For this review, take the finished solid that the model builds, in its own axes (mm). Give positions to 0.01 mm unless a question says otherwise; leave off trailing zeros. Order: outer loops, then holes, each group sorted by start corner. A loop starts at its lowest first (then second) coordinate and runs counter-clockwise, first axis right, second up. Notation, with made-up numbers: (88, 39.5) - (136, 39.5) arc R28 ccw to (136, 77.5) - close; hole circle Ø6 at (-21.75, 73). An arc over 180 degrees is marked (long way). Use a Markdown table: item, result. Add a question column.
1) We need section A-A on y = 2.05. Write out the cut boundary in (x, z), then the cut area to 4 significant figures.
2) Wall thickness on L1, parallel to Z at x = 0.4, y = 3.6; L2, parallel to Z at x = 2.8, y = 2.15; L3, parallel to Y at x = 2.05, z = 62: over which ranges is each line inside the solid? List them lowest first.
3) We need section B-B on x = 2.3. Write out the cut boundary in (y, z).
4) Clearance check with flat-ended pins moving along their axes: P1, Ø1, axis at x = 3, z = 26.5, coming from the -Y side; P2, Ø1.2, axis at x = 2.5, z = 129.5, coming from the +Y side; P3, Ø0.8, axis at x = 2.5, z = 130.5, coming from the -Y side; P4, Ø0.8, axis at y = 2, z = -1.5, coming from the -X side. State where each tip first meets the part, or that it passes through.
```python
from build123d import *

# Parameters (mm, degrees)
SKETCH1_W           = 5
SKETCH1_H           = 5
BOSS_EXTRUDE1_DEPTH = 127.3
SKETCH2_W           = 2.5
SKETCH2_H           = 2.5
BOSS_EXTRUDE2_DEPTH = 5
SKETCH3_W           = 2.5
SKETCH3_H           = 2.5
BOSS_EXTRUDE3_DEPTH = 5
SKETCH4_W           = 3
SKETCH4_H           = 3
CUT_EXTRUDE1_DEPTH  = 30


with BuildPart() as part:
    # Sketch1 → Boss-Extrude1 (new body)
    with BuildSketch(Plane.XY):
        with Locations((2.5, 2.5)):
            Rectangle(SKETCH1_W, SKETCH1_H)
    extrude(amount=BOSS_EXTRUDE1_DEPTH)

    # Sketch2 → Boss-Extrude2 (add)
    with BuildSketch(Plane(origin=(0, 0, 0), x_dir=(-1, 0, 0), z_dir=(0, 0, -1))):
        with Locations((-2.5, 2.5)):
            Rectangle(SKETCH2_W, SKETCH2_H)
    extrude(amount=BOSS_EXTRUDE2_DEPTH)

    # Sketch3 → Boss-Extrude3 (add)
    with BuildSketch(Plane.XY.offset(127.3)):
        with Locations((2.5, 2.5)):
            Rectangle(SKETCH3_W, SKETCH3_H)
    extrude(amount=BOSS_EXTRUDE3_DEPTH)

    # Sketch4 → Cut-Extrude1 (cut)
    with BuildSketch(Plane.ZY):
        with Locations((61.15, 2.5)):
            Rectangle(SKETCH4_W, SKETCH4_H)
    extrude(amount=-CUT_EXTRUDE1_DEPTH, mode=Mode.SUBTRACT)


solid = part.part
```
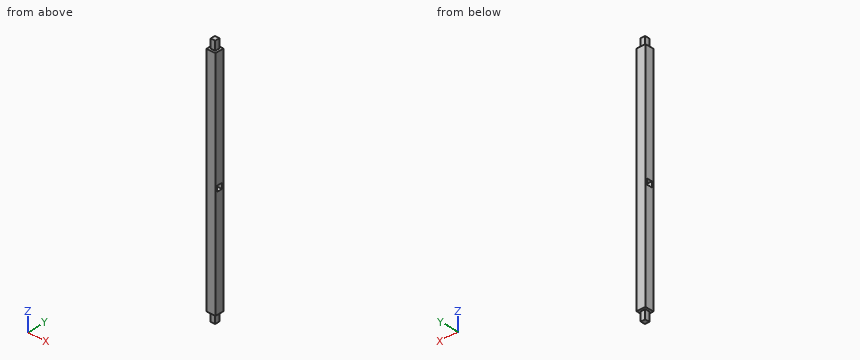
Checked values:
| question | item | result |
|---|---|---|
| 1 | outline | (0, 0) - (1.25, 0) - (1.25, -5) - (3.75, -5) - (3.75, 0) - (5, 0) - (5, 59.65) - (0, 59.65) - close; (0, 62.65) - (5, 62.65) - (5, 127.3) - (3.75, 127.3) - (3.75, 132.3) - (1.25, 132.3) - (1.25, 127.3) - (0, 127.3) - close |
| 1 | area | 646.5 mm² |
| 2 | L1 | 0 to 59.65, 62.65 to 127.3 |
| 2 | L2 | -5 to 59.65, 62.65 to 132.3 |
| 2 | L3 | 0 to 1, 4 to 5 |
| 3 | outline | (0, 0) - (1.25, 0) - (1.25, -5) - (3.75, -5) - (3.75, 0) - (5, 0) - (5, 127.3) - (3.75, 127.3) - (3.75, 132.3) - (1.25, 132.3) - (1.25, 127.3) - (0, 127.3) - close; hole (1, 59.65) - (4, 59.65) - (4, 62.65) - (1, 62.65) - close |
| 4 | P1 | y = 0 |
| 4 | P2 | y = 3.75 |
| 4 | P3 | y = 1.25 |
| 4 | P4 | x = 1.25 |
